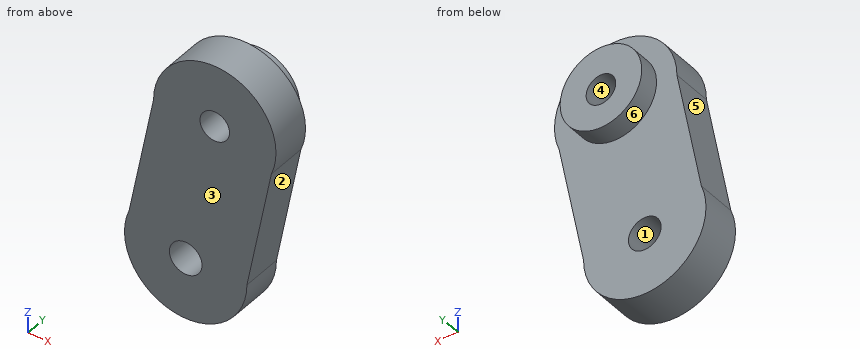
```python
from build123d import *

# Parameters (mm, degrees)
SKETCH1_R           = 1.6
SKETCH1_R_2         = 1.45
BOSS_EXTRUDE1_DEPTH = 4
SKETCH2_R           = 4
SKETCH2_R_2         = 1.45
BOSS_EXTRUDE2_DEPTH = 2


with BuildPart() as part:
    # Sketch1 → Boss-Extrude1 (new body)
    with BuildSketch(Plane(origin=(0, 0, 0), x_dir=(1, 0, 0), z_dir=(0, 1, 0))):
        with BuildLine():
            Line((-5.547666284, -2.285475619), (-3.15, -14.4))
            ThreePointArc((-3.15, -14.4), (4.014903922, -20.285830345), (8.397666284, -12.114524381))
            Line((8.397666284, -12.114524381), (6, 0))
            ThreePointArc((6, 0), (-1.164903922, 5.885830345), (-5.547666284, -2.285475619))
        make_face()
        with Locations(Location((0, 0, 0), (0, 0, 270))):
            Circle(SKETCH1_R, mode=Mode.SUBTRACT)
        with Locations(Location((2.85, -14.4, 0), (0, 0, 270))):
            Circle(SKETCH1_R_2, mode=Mode.SUBTRACT)
    extrude(amount=BOSS_EXTRUDE1_DEPTH)

    # Sketch2 → Boss-Extrude2 (add)
    with BuildSketch(Plane(origin=(0, 4, 0), x_dir=(1, 0, 0), z_dir=(0, 1, 0))):
        with Locations(Location((2.85, -14.602637459, 0), (0, 0, 270))):
            Circle(SKETCH2_R)
        with Locations(Location((2.85, -14.4, 0), (0, 0, 270))):
            Circle(SKETCH2_R_2, mode=Mode.SUBTRACT)
    extrude(amount=BOSS_EXTRUDE2_DEPTH)


solid = part.part
```
CAD build for the part. Positions are in the model's coordinates, mm. Face numbers are marked on the shaded views. A direction names the side the tool comes from. Coordinates: 2 decimals unless noted, no trailing zeros. Order: outer loops, then holes, each group sorted by start corner. A loop starts at its lowest first (then second) coordinate and runs counter-clockwise, first axis right, second up. Notation, with made-up numbers: (80, 77) -> (123, 77) arc R6 cw to (123, 86) -> close; hole circle Ø6 at (6.25, 35.5). An arc over 180 degrees is marked (long way). Use one line per item in the form item = value. Start each with the question number.
1) Pull direction Z, two halves, no side cores. Call the marked faces 1, 2, 3 and 4: +Z half, -Z half, draft (parallel to the pull), parting line (faces both ways), or undercut.
2) Band-saw the part on A-A on y = 2.75. Give the cut face in (x, z), then the cut area to 3 significant figures.
3) Band-saw the part on D-D on y = 4.8. Give the cut face in (x, z), then the cut area to 3 significant figures.
4) Drop flat-ended pins along their axis: pin 1 (2 mm diameter, centred on y = 1, z = 13, fed in from +X); pin 2 (1.5 mm diameter, centred on y = 5.5, z = 9, fed in from -X); pin 3 (2 mm diameter, centred on x = -0.5, z = 3.5, fed in from +Y); pin 4 (1 mm diameter, centred on x = -0.5, y = 5, fed in from -Z). Give the stop position or say it passes through.
5) Band-saw the part on B-B on x = -0.25. Give the cut face in (y, z), then the cut area to 3 significant figures.
6) Band-saw the part on C-C on z = -1. Give the cut face in (x, y), then the cut area to 3 significant figures.
7) Drill centre lines: L1, parallel to X at y = 4.3, z = 14.4; L2, parallel to Y at x = 5.5, z = 6.25; L3, parallel to X at y = 2.4, z = 13.75. Where is each one in solid material? Low to high. Write a range as [from, to].
8) Tool access for the marked faces 5 and 6: list every direction of +Z, -Z, +X, -X, +Y, -Y with a clear straight run to the whole face (end or side of a thin tool).
Entries:
q1.face_1 = undercut
q1.face_2 = -Z half
q1.face_3 = draft
q1.face_4 = undercut
q2.outline = (-5.55, 2.29) arc R6 ccw (long way) to (6, 0) -> (8.4, 12.11) arc R6 ccw (long way) to (-3.15, 14.4) -> close; hole circle Ø3.2 at (0, 0); hole circle Ø2.9 at (2.85, 14.4)
q2.area = 272 mm2
q3.outline = circle Ø8 at (2.85, 14.6); hole circle Ø2.9 at (2.85, 14.4)
q3.area = 43.7 mm2
q4.pin_1 = 8.84
q4.pin_2 = through
q4.pin_3 = 4
q4.pin_4 = 11.8
q5.outline = (0, -5.99) -> (4, -5.99) -> (4, -1.58) -> (0, -1.58) -> close; (0, 1.58) -> (4, 1.58) -> (4, 12.07) -> (6, 12.07) -> (6, 17.13) -> (4, 17.13) -> (4, 19.54) -> (0, 19.54) -> close
q5.area = 99.6 mm2
q6.outline = (-5.92, 0) -> (-1.25, 0) -> (-1.25, 4) -> (-5.92, 4) -> close; (1.25, 0) -> (5.92, 0) -> (5.92, 4) -> (1.25, 4) -> close
q6.area = 37.3 mm2
q7.L1 = [-1.14, 1.4], [4.3, 6.84]
q7.L2 = [0, 4]
q7.L3 = [-3.28, 1.55], [4.15, 8.81]
q8.face_5 = +Z, -X, +Y, -Y
q8.face_6 = +Y
